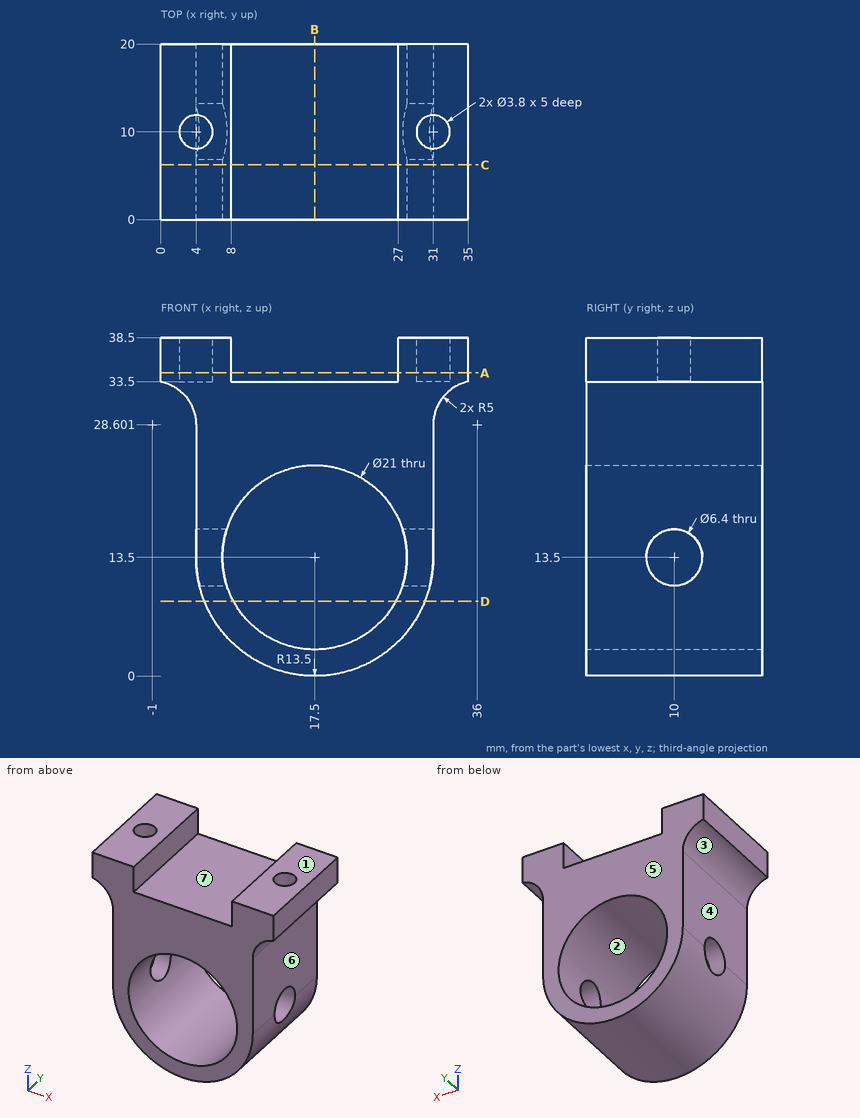
Geometry: see drawing. Coordinates: mm, zero at the bounding-box minimum. A direction names the side the tool comes from. Round coordinates to 2 decimals unless told otherwise and drop trailing zeros. Write each loop counter-clockwise with the first axis right and the second up, starting at its lowest first coordinate (ties: lowest second). Pieces come first, ordered by that corner, then holes. Notation, with made-up numbers: M -8.5,84.5 L 44.5,84.5 A23 ccw 44.5,115.5 Z; hole C 62,31.25 d8. An arc over 180 degrees is marked long. Answer in a Markdown table with one row per item. Add a question column.
(1) Cut plane A-A, the plane z = 34.5. Return the cut outline in (x, y), then the cut area to 3 significant figures.
(2) Reachability of the marked faces 5, 6 and 7 from +Z, -Z, +X, -X, +Y, -Y: full face, straight path, thin tool, end or side. Return the list, or none.
(3) Ray query, L1, parallel to X at y = 9.5, z = 36; L2, parallel to Y at x = 4, z = 37.4; L3, parallel to Y at x = 6.4, z = 13.5. Return the intervals inside material, ascending.
(4) Contact query for flat-ended pins moving along their axis: pin 1 (1.1 mm diameter, centred on x = 30.5, y = 9.5, fed in from +Z); pin 2 (7.5 mm diameter, centred on y = 12, z = 19, fed in from +X); pin 3 (7.5 mm diameter, centred on y = 10, z = 13.5, fed in from -X). Output: stop coordinate, or through.
(5) Cut plane D-D, the plane z = 8.5. Return the cut outline in (x, y), then the cut area to 3 significant figures.
(6) Draft query along Z for the marked faces 1, 2, 3 and 4. Return one class per face: pulls with the +Z half, pulls with the -Z half, needs draft (parallel to the pull), parting line crosses it, or undercut.
(7) Cut plane C-C, the plane y = 6.25. Return the cut outline in (x, z).
(8) Cut plane B-B, the plane x = 17.5. Return the cut outline in (y, z).
Established:
| question | item | result |
|---|---|---|
| 1 | outline | M 0,0 L 8,0 L 8,20 L 0,20 Z; M 27,0 L 35,0 L 35,20 L 27,20 Z; hole C 4,10 d3.8; hole C 31,10 d3.8 |
| 1 | area | 297 mm² |
| 2 | face 5 | +Z, -Z, +X, -X, +Y |
| 2 | face 6 | -Z, +X, +Y, -Y |
| 2 | face 7 | +Z, +Y, -Y |
| 3 | L1 | 0 to 2.17, 5.83 to 8, 27 to 29.17, 32.83 to 35 |
| 3 | L2 | 0 to 8.1, 11.9 to 20 |
| 3 | L3 | 0 to 6.8, 13.2 to 20 |
| 4 | pin 1 | z = 33.5 |
| 4 | pin 2 | x = 31 |
| 4 | pin 3 | x = 4 |
| 5 | outline | M 4.96,0 L 8.27,0 L 8.27,20 L 4.96,20 Z; M 26.73,0 L 30.04,0 L 30.04,20 L 26.73,20 Z |
| 5 | area | 132 mm² |
| 6 | face 1 | pulls with the +Z half |
| 6 | face 2 | undercut |
| 6 | face 3 | pulls with the -Z half |
| 6 | face 4 | needs draft |
| 7 | outline | M 0,33.5 A5 cw 4,28.6 L 4,13.5 A13.5 ccw 31,13.5 L 31,28.6 A5 cw 35,33.5 L 35,38.5 L 27,38.5 L 27,33.5 L 8,33.5 L 8,38.5 L 0,38.5 Z; hole C 17.5,13.5 d21 |
| 8 | outline | M 0,0 L 20,0 L 20,3 L 0,3 Z; M 0,24 L 20,24 L 20,33.5 L 0,33.5 Z |
